```python
from build123d import *

# Parameters (mm, degrees)
CUT_EXTRUDE_1_DEPTH = 2.5
FILLET_1_R          = 0.3
CHAMFER_1_SIZE      = 1.6


with BuildPart() as part:
    # Эскиз1 → Повернуть1 (revolve)
    with BuildSketch(Plane.XY):
        Polygon((0, 0), (0, 6.5), (8, 6.5), (8, 4), (48, 4), (48, 0), align=None)
    revolve(axis=Axis((48, 0, 0), (-1, 0, 0)))

    # Эскиз2 → Вырез-Вытянуть1 (cut)
    with BuildSketch(Plane.ZY):
        Polygon((-1.732050808, 3), (-3.464101615, 0), (-1.732050808, -3), (1.732050808, -3), (3.464101615, 0), (1.732050808, 3), align=None)
    extrude(amount=-CUT_EXTRUDE_1_DEPTH, mode=Mode.SUBTRACT)

    # Скругление1
    fillet_1_edges = [part.edges().sort_by_distance(p)[0] for p in [
        (8, -4, 0),
        (0, -6.5, 0),
    ]]
    fillet(fillet_1_edges, radius=FILLET_1_R)

    # Фаска1
    chamfer_1_edges = [part.edges().sort_by_distance(p)[0] for p in [
        (48, -4, 0),
    ]]
    chamfer(chamfer_1_edges, length=CHAMFER_1_SIZE)


solid = part.part
```
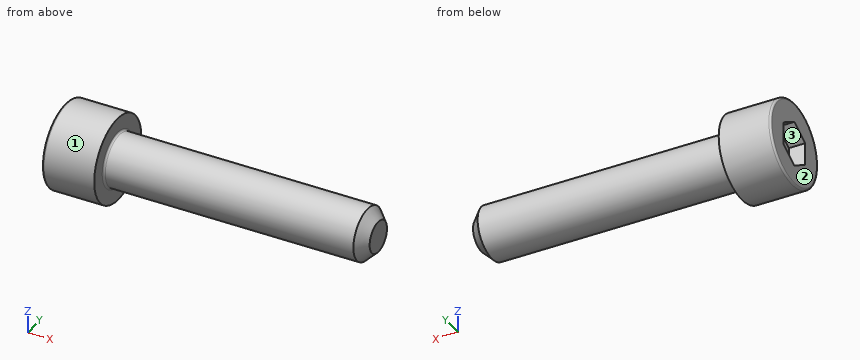
Source: CAD feature listing. Evaluate the final solid. Frame: model axes, mm. Face numbers are marked on the shaded views. Give positions to 0.01 mm unless a question says otherwise; leave off trailing zeros. Order: outer loops, then holes, each group sorted by start corner. A loop starts at its lowest first (then second) coordinate and runs counter-clockwise, first axis right, second up.
(1) Pull-direction query (Y, two-part tool) for the marked faces 1, 2 and 3; classes: +Y half, -Y half, draft (parallel to the pull), parting line (faces both ways), or undercut.
(2) Section query A-A (z = 0). Return the cut outline in (x, y).
(3) Section query B-B (x = 33). Return the cut outline in (y, z), plus the area to 3 significant figures.
(4) Material intervals for line 1 along X through (y, z) = (1.75, 0); line 2 along X through (y, z) = (5.75, -0.5); line 3 along Y through (x, z) = (22.5, 2), sorted ascending.
(5) Contact query for flat-ended pins moving along their axis: P1, Ø4, axis at x = 19, y = 1.5, coming from the -Z side; P2, Ø4, axis at x = 12.5, y = -3.5, coming from the +Z side; P3, Ø1.8, axis at y = 0.5, z = 0.5, coming from the -X side. Output: stop coordinate, or through.
Outcome:
1. face 1: parting line
1. face 2: draft
1. face 3: undercut
2. outline: (0, -6.2) arc R0.3 ccw to (0.3, -6.5) - (8, -6.5) - (8, -4.3) arc R0.3 cw to (8.3, -4) - (46.4, -4) - (48, -2.4) - (48, 2.4) - (46.4, 4) - (8.3, 4) arc R0.3 cw to (8, 4.3) - (8, 6.5) - (0.3, 6.5) arc R0.3 ccw to (0, 6.2) - (0, 3) - (2.5, 3) - (2.5, -3) - (0, -3) - close
3. outline: circle Ø8 at (0, 0)
3. area: 50.3 mm2
4. line 1: x = 2.5 to 48
4. line 2: x = 0 to 8
4. line 3: y = -3.46 to 3.46
5. P1: stops at z = -4
5. P2: stops at z = 3.71
5. P3: stops at x = 2.5
